Could you check a few things on this model? Use its own coordinates, in mm. A direction names the side the tool comes from. Give positions to 0.01 mm unless a question says otherwise; leave off trailing zeros. Loops run counter-clockwise (first coordinate to the right, second up) from the corner with the lowest first, then second, coordinate; pieces in that order, holes last. Notation, with made-up numbers: M 10.25,62.5 L 59.25,62.5 A25 cw 59.25,87.5 Z; hole C 81.25,61 d9. An arc over 180 degrees is marked long. Return JSON: item names as keys, results as strings. Group by question number.
1. If we section it at B-B (x = 14.5): Write out the boundary of the cut face in (y, z) (3 decimals), plus the area to 3 significant figures.
2. If we section it at A-A (y = 279.4): Write out the boundary of the cut face in (x, z) (3 decimals).
3. For pin 1 (7.5 mm diameter, centred on x = 0, y = 177.8, fed in from -Z); pin 2 (1.5 mm diameter, centred on x = -1, z = -6, fed in from -Y), each with a flat end and sliding along its axis, tell me the tip position at first contact or that it passes through.
4. If we mould it in two halves opening along Y, with no side actions, what happens to faces 1 (the cylindrical face through (0.8, 260.3, -14.6)), 2 (the flat face through (-1, 304.8, 0)), 3 (the flat face through (38.1, 150, 0))? For each: +Y half, -Y half, draft (parallel to the pull), parting line (faces both ways), or undercut.
5. Please list where these lines run through material, in increasing order: line 1 (Z direction, x = -13, y = 61.5) (3 decimals); line 2 (X direction, y = 176.5, z = -10.5); line 3 (X direction, y = 279.4, z = -14.2).
6. For faces 4 (the cylindrical face through (-3.414, 208.554, 14.587)), 5 (the flat face through (35.56, 149, 0)), which set-ups out of +Z, -Z, +X, -X, +Y, -Y let a thin tool reach every point of the face, with its end or its side?
7. If we section it at D-D (x = 0): State how many separate pieces and enclosed holes the cut face has, plus the area to 3 significant figures.
8. If we section it at C-C (z = 7.5): Write out the boundary of the cut face in (x, y), plus the area to 3 significant figures.
```python
from build123d import *

# Parameters (mm, degrees)
F0_W     = 76.2
F0_H     = 31.75
F1_DEPTH = 304.8
F2_T     = -2.54
F4_D     = 12.7


with BuildPart() as f1:
    # F0 (on Front) → F1 (new body)
    with BuildSketch(Plane.XZ):
        Rectangle(F0_W, F0_H)
    extrude(amount=-F1_DEPTH)

    # F2
    f2_openings = [f1.faces().sort_by_distance(p)[0] for p in [
        (0, 0, 0),
    ]]
    offset(amount=F2_T, openings=f2_openings)

    # F4 (through all)
    with Locations(Plane.XY.offset(15.875)):
        with Locations((0, 279.4), (0, 254), (0, 228.6), (0, 203.2), (0, 177.8), (0, 152.4), (0, 127), (0, 101.6), (0, 76.2), (0, 25.4), (0, 50.8)):
            Hole(F4_D / 2)


solid = f1.part
```
Answer:
{
 "1": {"outline": "M 0,-15.875 L 304.8,-15.875 L 304.8,15.875 L 0,15.875 L 0,13.335 L 302.26,13.335 L 302.26,-13.335 L 0,-13.335 Z", "area": "1,620 mm²"},
 "2": {"outline": "M -38.1,-15.875 L -6.35,-15.875 L -6.35,-13.335 L -35.56,-13.335 L -35.56,13.335 L -6.35,13.335 L -6.35,15.875 L -38.1,15.875 Z; M 6.35,-15.875 L 38.1,-15.875 L 38.1,15.875 L 6.35,15.875 L 6.35,13.335 L 35.56,13.335 L 35.56,-13.335 L 6.35,-13.335 Z"},
 "3": {"pin 1": "passes through", "pin 2": "stops at y = 302.26"},
 "4": {"face 1": "undercut", "face 2": "+Y half", "face 3": "draft"},
 "5": {"line 1": "z = -15.875 to -13.335, 13.335 to 15.875", "line 2": "x = -38.1 to -35.56, 35.56 to 38.1", "line 3": "x = -38.1 to -6.35, 6.35 to 38.1"},
 "6": {"face 4": "+Z, -Z", "face 5": "-Y"},
 "7": {"separate pieces": "23", "enclosed holes": "0", "area": "906 mm²"},
 "8": {"outline": "M -38.1,0 L -35.56,0 L -35.56,302.26 L 35.56,302.26 L 35.56,0 L 38.1,0 L 38.1,304.8 L -38.1,304.8 Z", "area": "1,730 mm²"}
}
